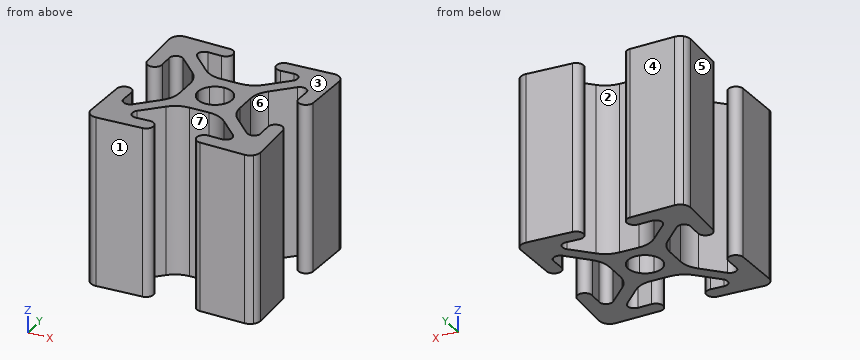
from build123d import *

# Parameters (mm, degrees)
EXTRUDE1_DEPTH = 25.4


with BuildPart() as part:
    # Sketch1 → Extrude1 (new body)
    with BuildSketch(Plane.XY):
        with BuildLine():
            Line((11.119216576, 12.698941773), (4.314458822, 12.445223967))
            ThreePointArc((4.314458822, 12.445223967), (3.239276033, 11.286758822), (4.397741178, 10.211576033))
            Line((4.397741178, 10.211576033), (6.439144384, 10.287690476))
            ThreePointArc((6.439144384, 10.287690476), (7.408254029, 9.678624879), (7.19542049, 8.553975471))
            Line((7.19542049, 8.553975471), (4.34026306, 5.698818041))
            ThreePointArc((4.34026306, 5.698818041), (3.02180657, 4.81785358), (1.466581101, 4.5085))
            Line((1.466581101, 4.5085), (0, 4.5085))
            Line((0, 4.5085), (-1.466581101, 4.5085))
            ThreePointArc((-1.466581101, 4.5085), (-3.02180657, 4.81785358), (-4.34026306, 5.698818041))
            Line((-4.34026306, 5.698818041), (-7.19542049, 8.553975471))
            ThreePointArc((-7.19542049, 8.553975471), (-7.408254029, 9.678624879), (-6.439144384, 10.287690476))
            Line((-6.439144384, 10.287690476), (-4.397741178, 10.211576033))
            ThreePointArc((-4.397741178, 10.211576033), (-3.239276033, 11.286758822), (-4.314458822, 12.445223967))
            Line((-4.314458822, 12.445223967), (-11.119216576, 12.698941773))
            ThreePointArc((-11.119216576, 12.698941773), (-11.732873224, 12.594614892), (-12.253630735, 12.253630735))
            ThreePointArc((-12.253630735, 12.253630735), (-12.594614892, 11.732873224), (-12.698941773, 11.119216576))
            Line((-12.698941773, 11.119216576), (-12.445223967, 4.314458822))
            ThreePointArc((-12.445223967, 4.314458822), (-11.286758822, 3.239276033), (-10.211576033, 4.397741178))
            Line((-10.211576033, 4.397741178), (-10.287690476, 6.439144384))
            ThreePointArc((-10.287690476, 6.439144384), (-9.678624879, 7.408254029), (-8.553975471, 7.19542049))
            Line((-8.553975471, 7.19542049), (-5.698818041, 4.34026306))
            ThreePointArc((-5.698818041, 4.34026306), (-4.81785358, 3.02180657), (-4.5085, 1.466581101))
            Line((-4.5085, 1.466581101), (-4.5085, 0))
            Line((-4.5085, 0), (-4.5085, -1.466581101))
            ThreePointArc((-4.5085, -1.466581101), (-4.81785358, -3.02180657), (-5.698818041, -4.34026306))
            Line((-5.698818041, -4.34026306), (-8.553975471, -7.19542049))
            ThreePointArc((-8.553975471, -7.19542049), (-9.678624879, -7.408254029), (-10.287690476, -6.439144384))
            Line((-10.287690476, -6.439144384), (-10.211576033, -4.397741178))
            ThreePointArc((-10.211576033, -4.397741178), (-11.286758822, -3.239276033), (-12.445223967, -4.314458822))
            Line((-12.445223967, -4.314458822), (-12.698941773, -11.119216576))
            ThreePointArc((-12.698941773, -11.119216576), (-12.594614892, -11.732873224), (-12.253630735, -12.253630735))
            ThreePointArc((-12.253630735, -12.253630735), (-11.732873224, -12.594614892), (-11.119216576, -12.698941773))
            Line((-11.119216576, -12.698941773), (-4.314458822, -12.445223967))
            ThreePointArc((-4.314458822, -12.445223967), (-3.239276033, -11.286758822), (-4.397741178, -10.211576033))
            Line((-4.397741178, -10.211576033), (-6.439144384, -10.287690476))
            ThreePointArc((-6.439144384, -10.287690476), (-7.408254029, -9.678624879), (-7.19542049, -8.553975471))
            Line((-7.19542049, -8.553975471), (-4.34026306, -5.698818041))
            ThreePointArc((-4.34026306, -5.698818041), (-3.02180657, -4.81785358), (-1.466581101, -4.5085))
            Line((-1.466581101, -4.5085), (0, -4.5085))
            Line((0, -4.5085), (1.466581101, -4.5085))
            ThreePointArc((1.466581101, -4.5085), (3.02180657, -4.81785358), (4.34026306, -5.698818041))
            Line((4.34026306, -5.698818041), (7.19542049, -8.553975471))
            ThreePointArc((7.19542049, -8.553975471), (7.408254029, -9.678624879), (6.439144384, -10.287690476))
            Line((6.439144384, -10.287690476), (4.397741178, -10.211576033))
            ThreePointArc((4.397741178, -10.211576033), (3.239276033, -11.286758822), (4.314458822, -12.445223967))
            Line((4.314458822, -12.445223967), (11.119216576, -12.698941773))
            ThreePointArc((11.119216576, -12.698941773), (11.732873224, -12.594614892), (12.253630735, -12.253630735))
            ThreePointArc((12.253630735, -12.253630735), (12.594614892, -11.732873224), (12.698941773, -11.119216576))
            Line((12.698941773, -11.119216576), (12.445223967, -4.314458822))
            ThreePointArc((12.445223967, -4.314458822), (11.286758822, -3.239276033), (10.211576033, -4.397741178))
            Line((10.211576033, -4.397741178), (10.287690476, -6.439144384))
            ThreePointArc((10.287690476, -6.439144384), (9.678624879, -7.408254029), (8.553975471, -7.19542049))
            Line((8.553975471, -7.19542049), (5.698818041, -4.34026306))
            ThreePointArc((5.698818041, -4.34026306), (4.81785358, -3.02180657), (4.5085, -1.466581101))
            Line((4.5085, -1.466581101), (4.5085, 0))
            Line((4.5085, 0), (4.5085, 1.466581101))
            ThreePointArc((4.5085, 1.466581101), (4.81785358, 3.02180657), (5.698818041, 4.34026306))
            Line((5.698818041, 4.34026306), (8.553975471, 7.19542049))
            ThreePointArc((8.553975471, 7.19542049), (9.678624879, 7.408254029), (10.287690476, 6.439144384))
            Line((10.287690476, 6.439144384), (10.211576033, 4.397741178))
            ThreePointArc((10.211576033, 4.397741178), (11.286758822, 3.239276033), (12.445223967, 4.314458822))
            Line((12.445223967, 4.314458822), (12.698941773, 11.119216576))
            ThreePointArc((12.698941773, 11.119216576), (12.594614892, 11.732873224), (12.253630735, 12.253630735))
            ThreePointArc((12.253630735, 12.253630735), (11.732873224, 12.594614892), (11.119216576, 12.698941773))
        make_face()
        with BuildLine():
            ThreePointArc((1.80503148, 1.80503148), (0.976875998, 2.358387283), (0, 2.5527))
            ThreePointArc((0, 2.5527), (-0.976875998, 2.358387283), (-1.80503148, 1.80503148))
            ThreePointArc((-1.80503148, 1.80503148), (-2.358387283, 0.976875998), (-2.5527, 0))
            ThreePointArc((-2.5527, 0), (-2.358387283, -0.976875998), (-1.80503148, -1.80503148))
            ThreePointArc((-1.80503148, -1.80503148), (-0.976875998, -2.358387283), (0, -2.5527))
            ThreePointArc((0, -2.5527), (0.976875998, -2.358387283), (1.80503148, -1.80503148))
            ThreePointArc((1.80503148, -1.80503148), (2.358387283, -0.976875998), (2.5527, 0))
            ThreePointArc((2.5527, 0), (2.358387283, 0.976875998), (1.80503148, 1.80503148))
        make_face(mode=Mode.SUBTRACT)
    extrude(amount=EXTRUDE1_DEPTH)


solid = part.part
Here's how the part is built. I have some questions about the finished solid (model axes, mm). Face numbers are marked on the shaded views. A direction names the side the tool comes from. Coordinates: 2 decimals unless noted, no trailing zeros. Loops run counter-clockwise (first coordinate to the right, second up) from the corner with the lowest first, then second, coordinate; pieces in that order, holes last.
1. Imagine slicing it at A-A, the plane x = -9. Please give me the cut outline in (y, z).
2. If we mould it in two halves opening along Y, with no side actions, what happens to the marked faces 1, 2, 3 and 4? For each: pulls with the +Y half, pulls with the -Y half, needs draft (parallel to the pull), parting line crosses it, or undercut.
3. Imagine slicing it at B-B, the plane y = -0.75. Please give me the cut outline in (x, z).
4. For the marked faces 5, 6 and 7, which set-ups out of +Z, -Z, +X, -X, +Y, -Y let a thin tool reach every point of the face, with its end or its side?
5. I need wall thicknesses on L1, parallel to Y at x = -7.25, z = 8; L2, parallel to X at y = -7, z = 3; L3, parallel to Y at x = 5.5, z = 5. Which ranges of each line are inside material? Lowest first, please.
6. For P1, Ø2, axis at y = -5, z = 11, coming from the -X side; P2, Ø2.5, axis at y = -0.5, z = 7.5, coming from the +X side; P3, Ø1.5, axis at x = -6.5, y = -3, coming from the +Z side; P4, Ø0.9, axis at x = -0.5, z = 17, coming from the +Y side, each with a flat end and sliding along its axis, tell me the tip position at first contact or that it passes through.
Taken from the geometry:
1. outline: (-12.62, 0) - (-7.46, 0) - (-7.46, 25.4) - (-12.62, 25.4) - close; (7.46, 0) - (12.62, 0) - (12.62, 25.4) - (7.46, 25.4) - close
2. face 1: pulls with the -Y half
2. face 2: undercut
2. face 3: needs draft
2. face 4: pulls with the +Y half
3. outline: (-4.51, 0) - (-2.44, 0) - (-2.44, 25.4) - (-4.51, 25.4) - close; (2.44, 0) - (4.51, 0) - (4.51, 25.4) - (2.44, 25.4) - close
4. face 5: +Z, -Z, -X
4. face 6: +Z, -Z
4. face 7: +Z, -Z, -Y
5. L1: y = -12.55 to -9.93, -8.61 to -5.89, 5.89 to 8.61, 9.93 to 12.55
5. L2: x = -12.55 to -10.14, -8.36 to -5.64, 5.64 to 8.36, 10.14 to 12.55
5. L3: y = -12.49 to -10.25, -6.86 to -4.13, 4.13 to 6.86, 10.25 to 12.49
6. P1: stops at x = -12.51
6. P2: stops at x = 4.52
6. P3: passes through
6. P4: stops at y = 4.51
